```python
from build123d import *

# Parameters (mm, degrees)
SKETCH_1_W          = 100
SKETCH_1_H          = 100
EXTRUDE_1_DEPTH     = 2
SKETCH_2_W          = 6
SKETCH_2_H          = 12
EXTRUDE_2_DEPTH     = 10
SKETCH_3_R          = 3.725
CUT_EXTRUDE_1_DEPTH = 142.929559994
SKETCH_4_R          = 6
EXTRUDE_3_DEPTH     = 5
SKETCH_5_R          = 3.75
CUT_EXTRUDE_2_DEPTH = 142.594491418
SKETCH_6_W          = 100
SKETCH_6_H          = 19
CUT_EXTRUDE_3_DEPTH = 142.774468788
CUT_EXTRUDE_4_DEPTH = 130.077496102
FILLET_1_R          = 6
CUT_EXTRUDE_6_DEPTH = 130.077496102
FILLET_2_R          = 2
FILLET_3_R          = 2


# Some blends are built 0.0001 mm under size
with BuildPart() as part:
    # 草图1 → 凸台-拉伸1 (new body)
    with BuildSketch(Plane(origin=(0, 0, 0), x_dir=(1, 0, 0), z_dir=(0, 1, 0))):
        with Locations((50, -50)):
            Rectangle(SKETCH_1_W, SKETCH_1_H)
    extrude(amount=EXTRUDE_1_DEPTH)

    # 草图2 → 凸台-拉伸2 (add)
    with BuildSketch(Plane(origin=(0, 2, 0), x_dir=(1, 0, 0), z_dir=(0, 1, 0))):
        with Locations((97, -25)):
            Rectangle(SKETCH_2_W, SKETCH_2_H)
        with Locations((97, -75)):
            Rectangle(SKETCH_2_W, SKETCH_2_H)
    extrude(amount=EXTRUDE_2_DEPTH)

    # 草图3 → 切除-拉伸1 (cut, through all)
    with BuildSketch(Plane(origin=(100, 0, 0), x_dir=(0, 0, -1), z_dir=(1, 0, 0))):
        with Locations((-25, 6)):
            Circle(SKETCH_3_R)
        with Locations((-75, 6)):
            Circle(SKETCH_3_R)
    extrude(amount=-CUT_EXTRUDE_1_DEPTH, mode=Mode.SUBTRACT)

    # 草图4 → 凸台-拉伸3 (add)
    with BuildSketch(Plane(origin=(0, 2, 0), x_dir=(1, 0, 0), z_dir=(0, 1, 0))):
        with Locations(Location((50, -50, 0), (0, 0, 270))):
            Circle(SKETCH_4_R)
    extrude(amount=EXTRUDE_3_DEPTH)

    # 草图5 → 切除-拉伸2 (cut, through all)
    with BuildSketch(Plane(origin=(0, 7, 0), x_dir=(1, 0, 0), z_dir=(0, 1, 0))):
        with Locations(Location((50, -50, 0), (0, 0, 270))):
            Circle(SKETCH_5_R)
    extrude(amount=-CUT_EXTRUDE_2_DEPTH, mode=Mode.SUBTRACT)

    # 草图6 → 切除-拉伸3 (cut, through all)
    with BuildSketch(Plane(origin=(0, 2, 0), x_dir=(1, 0, 0), z_dir=(0, 1, 0))):
        with Locations((50, -90.5)):
            Rectangle(SKETCH_6_W, SKETCH_6_H)
        with Locations((50, -9.5)):
            Rectangle(SKETCH_6_W, SKETCH_6_H)
    extrude(amount=-CUT_EXTRUDE_3_DEPTH, mode=Mode.SUBTRACT)

    # 草图7 → 切除-拉伸4 (cut, through all)
    with BuildSketch(Plane(origin=(0, 2, 0), x_dir=(1, 0, 0), z_dir=(0, 1, 0))):
        with BuildLine():
            Line((55.73131114, -53.066279932), (94, -69))
            Line((94, -69), (94, -31))
            Line((94, -31), (55.73131114, -46.933720068))
            ThreePointArc((55.73131114, -46.933720068), (56.304899777, -48.41941821), (56.5, -50))
            ThreePointArc((56.5, -50), (56.304899777, -51.58058179), (55.73131114, -53.066279932))
        make_face()
        Polygon((0, -19), (53.212773637, -41.880071279), (94, -19), align=None)
        with BuildLine():
            Line((4, -75.253806127), (47.820913419, -56.123853499))
            ThreePointArc((47.820913419, -56.123853499), (43.5, -50), (47.820913419, -43.876146501))
            Line((47.820913419, -43.876146501), (4, -24.746193873))
            Line((4, -24.746193873), (4, -75.253806127))
        make_face()
        Polygon((94, -81), (53.212773637, -58.119928721), (0, -81), align=None)
    extrude(amount=-CUT_EXTRUDE_4_DEPTH, mode=Mode.SUBTRACT)

    # 圆角1
    fillet_1_edges = [part.edges().sort_by_distance(p)[0] for p in [
        (97, 12, 81),
        (97, 12, 69),
        (97, 12, 31),
        (97, 12, 19),
    ]]
    fillet(fillet_1_edges, radius=FILLET_1_R - 0.0001)  # a hair under: the kernel refuses the full size

    # 草图8 → 切除-拉伸6 (cut, through all)
    with BuildSketch(Plane(origin=(0, 2, 0), x_dir=(1, 0, 0), z_dir=(0, 1, 0))):
        Polygon((91.5, -23.268889447), (91.5, -29.332868234), (56.926900292, -43.727876504), (56.51218358, -42.895713945), align=None)
        Polygon((91.5, -70.667131766), (91.5, -76.731110553), (56.51218358, -57.104286055), (56.926900292, -56.272123496), align=None)
    extrude(amount=-CUT_EXTRUDE_6_DEPTH, mode=Mode.SUBTRACT)

    # 圆角2
    fillet_2_edges = [part.edges().sort_by_distance(p)[0] for p in [
        (47.820913419, 1, 43.876146501),
        (47.820913419, 1, 56.123853499),
        (55.73131114, 1, 53.066279932),
        (55.73131114, 1, 46.933720068),
    ]]
    fillet(fillet_2_edges, radius=FILLET_2_R)

    # 圆角3
    # the kernel refuses this fillet: 2 mm, written as the material it adds along each edge
    with BuildSketch(Plane(origin=(4, 2, 75.253806127), x_dir=(0, 0, -1), z_dir=(0, -1, 0)), Plane(origin=(4, 2, 24.746193873), x_dir=(0.9164772733710811, 0, 0.4000867498359684), z_dir=(0, -1, 0))) as fillet_3_piece_1:
        with BuildLine():
            CenterArc((FILLET_3_R * 1.52768299937, FILLET_3_R), FILLET_3_R, 156.416398259, 113.583601741)
            Line((FILLET_3_R * 0.611205725997, FILLET_3_R * 1.40008674984), (0, 0))
            Line((0, 0), (FILLET_3_R * 1.52768299937, 0))
        make_face()
    extrude(amount=2)
    with BuildSketch(Plane(origin=(53.212773637, 2, 58.119928721), x_dir=(-0.9186780925924477, 0, 0.39500704068497583), z_dir=(0, -1, 0))) as fillet_3_piece_2:
        with BuildLine():
            CenterArc((FILLET_3_R * 0.493765794488, -FILLET_3_R), FILLET_3_R, 90, 52.557168538)
            Line((-FILLET_3_R * 0.300194560291, -FILLET_3_R * 0.39203046537), (0, 0))
            Line((0, 0), (FILLET_3_R * 0.493765794488, 0))
        make_face()
    extrude(amount=2)
    with BuildSketch(Plane(origin=(53.212773637, 2, 41.880071279), x_dir=(-0.918678092592448, 0, -0.395007040684975), z_dir=(0, -1, 0))) as fillet_3_piece_3:
        with BuildLine():
            CenterArc((FILLET_3_R * 0.493765794488, FILLET_3_R), FILLET_3_R, 217.442831462, 52.557168538)
            Line((-FILLET_3_R * 0.300194560291, FILLET_3_R * 0.39203046537), (0, 0))
            Line((0, 0), (FILLET_3_R * 0.493765794488, 0))
        make_face()
    extrude(amount=2)
    with BuildSketch(Plane(origin=(91.5, 2, 23.268889447), x_dir=(-0.8721482225909527, 0, 0.48924173762204914), z_dir=(0, -1, 0))) as fillet_3_piece_4:
        with BuildLine():
            CenterArc((FILLET_3_R * 1.70755577899, -FILLET_3_R), FILLET_3_R, 90, 119.290755367)
            Line((FILLET_3_R * 0.8354075564, -FILLET_3_R * 1.48924173762), (0, 0))
            Line((0, 0), (FILLET_3_R * 1.70755577899, 0))
        make_face()
    extrude(amount=2)
    with BuildSketch(Plane(origin=(91.5, 2, 29.332868234), x_dir=(-0.9231759584436576, 0, 0.38437761348917576), z_dir=(0, -1, 0))) as fillet_3_piece_5:
        with BuildLine():
            CenterArc((FILLET_3_R * 0.666852706551, FILLET_3_R), FILLET_3_R, 202.605107184, 67.394892816)
            Line((-FILLET_3_R * 0.256323251893, FILLET_3_R * 0.615622386511), (0, 0))
            Line((0, 0), (FILLET_3_R * 0.666852706551, 0))
        make_face()
    extrude(amount=2)
    with BuildSketch(Plane(origin=(91.5, 2, 70.667131766), x_dir=(-0.923175958443657, 0, -0.38437761348917726), z_dir=(0, -1, 0))) as fillet_3_piece_6:
        with BuildLine():
            CenterArc((FILLET_3_R * 0.666852706551, -FILLET_3_R), FILLET_3_R, 90, 67.394892816)
            Line((-FILLET_3_R * 0.256323251893, -FILLET_3_R * 0.615622386511), (0, 0))
            Line((0, 0), (FILLET_3_R * 0.666852706551, 0))
        make_face()
    extrude(amount=2)
    with BuildSketch(Plane(origin=(91.5, 2, 76.731110553), x_dir=(-0.8721482225909533, 0, -0.4892417376220482), z_dir=(0, -1, 0))) as fillet_3_piece_7:
        with BuildLine():
            CenterArc((FILLET_3_R * 1.70755577899, FILLET_3_R), FILLET_3_R, 150.709244633, 119.290755367)
            Line((FILLET_3_R * 0.8354075564, FILLET_3_R * 1.48924173762), (0, 0))
            Line((0, 0), (FILLET_3_R * 1.70755577899, 0))
        make_face()
    extrude(amount=2)
    with BuildSketch(Plane(origin=(94, 2, 31), x_dir=(0, 0, 1), z_dir=(0, -1, 0)), Plane(origin=(94, 2, 69), x_dir=(-0.9231759584436573, 0, -0.3843776134891767), z_dir=(0, -1, 0))) as fillet_3_piece_8:
        with BuildLine():
            CenterArc((FILLET_3_R * 1.49958152704, FILLET_3_R), FILLET_3_R, 157.394892816, 112.605107184)
            Line((FILLET_3_R * 0.576405568596, FILLET_3_R * 1.38437761349), (0, 0))
            Line((0, 0), (FILLET_3_R * 1.49958152704, 0))
        make_face()
    extrude(amount=2)
    # the kernel refuses this fillet: 2 mm, written as the material it takes off along each edge
    with BuildSketch(Plane(origin=(0, 9.592469288, 81), x_dir=(0.9186780925924475, 0, -0.3950070406849762), z_dir=(0, -1, 0)), Plane(origin=(0, 9.592469288, 19), x_dir=(0, 0, 1), z_dir=(0, -1, 0))) as fillet_3_2_piece_1:
        with BuildLine():
            CenterArc((FILLET_3_R * 1.51849385757, -FILLET_3_R), FILLET_3_R, 90, 113.266413172)
            Line((FILLET_3_R * 0.599815764977, -FILLET_3_R * 1.39500704068), (0, 0))
            Line((0, 0), (FILLET_3_R * 1.51849385757, 0))
        make_face()
    extrude(amount=17.184938576, mode=Mode.SUBTRACT)


solid = part.part
```
Work out the finished part from the listing and answer in its coordinate system (mm). A direction names the side the tool comes from. Give positions to 0.01 mm unless a question says otherwise; leave off trailing zeros. Loops run counter-clockwise (first coordinate to the right, second up) from the corner with the lowest first, then second, coordinate; pieces in that order, holes last. Notation, with made-up numbers: (49, -17.75) -> (89, -17.75) arc R28 ccw to (89, 15.25) -> close; hole circle Ø4 at (-11.75, 71). An arc over 180 degrees is marked (long way). Put each result on its own line as item: value. Start each with the question number.
Item 1: Each of these flat-tipped pins is pushed along its axis until it touches: P1, Ø10, axis at x = 22, z = 28.5, coming from the +Y side; P2, Ø6.5, axis at y = 6, z = 75, coming from the +X side; P3, Ø13, axis at x = 49, z = 52, coming from the +Y side; P4, Ø12, axis at x = 50, z = 50, coming from the -Y side. Where does it stop, or does it pass through?
Item 2: Find the intervals of material crossed by L1, parallel to X at y = 5.25, z = 50; L2, parallel to Y at x = 98.35, z = 75 (3 decimals); L3, parallel to X at y = 1.75, z = 67.5, in increasing order. Write a range as [from, to].
Item 3: The part is cut by section D-D (x = 27). Give the vertices of the cut face in (y, z), then the cut area to 3 significant figures.
Item 4: The part is cut by section B-B (y = 10.75). Give the vertices of the cut face in (x, z), then the cut area to 3 significant figures.
Item 5: The mould has two halves that part along X. Classify faces 1 (the face through (50, 4, 44)), 2 (the face through (27.89, 1.01, 69.01)), 3 (the face through (57, 2, 46)): released by +X, released by -X, zero draft, split by the parting line, or undercut.
Item 6: Which of the six approach directions +Z, -Z, +X, -X, +Y, -Y give full straight-line access (tool end or side, diameter ignored) to faces 4 (the face through (45.673, 0.986, 56.173)), 5 (the face through (94, 10, 25)), 6 (the face through (97, 4, 69))?
Item 7: The part is cut by section A-A (x = 48.5). Give the vertices of the cut face in (y, z), then the cut area to 3 significant figures.
Item 8: The part is cut by section C-C (x = 59). Give the vertices of the cut face in (y, z), then the cut area to 3 significant figures.
Answers below:
1. P1: y = 2
1. P2: through
1. P3: y = 7
1. P4: y = 0
2. L1: [44, 46.25], [53.75, 56]
2. L2: [0, 2.275], [9.725, 12]
2. L3: [0, 4], [21.76, 31.4], [69.93, 75.04], [83.89, 90.4], [93.32, 100]
3. outline: (0, 30.61) -> (2, 30.61) -> (2, 34.79) -> (0, 34.79) -> close; (0, 65.21) -> (2, 65.21) -> (2, 69.39) -> (0, 69.39) -> close
3. area: 16.7 mm2
4. outline: (94, 21.33) -> (100, 21.33) -> (100, 28.67) -> (94, 28.67) -> close; (94, 71.33) -> (100, 71.33) -> (100, 78.67) -> (94, 78.67) -> close
4. area: 88.0 mm2
5. face 1: split by the parting line
5. face 2: undercut
5. face 3: zero draft
6. face 4: +Y, -Y
6. face 5: +Z, -Z, -X, +Y
6. face 6: +X, -X, +Y
7. outline: (0, 39.85) -> (2, 39.85) -> (2, 44.19) -> (7, 44.19) -> (7, 46.56) -> (0, 46.56) -> close; (0, 53.44) -> (7, 53.44) -> (7, 55.81) -> (2, 55.81) -> (2, 60.15) -> (0, 60.15) -> close
7. area: 50.6 mm2
8. outline: (0, 38.63) -> (2, 38.63) -> (2, 41.5) -> (0, 41.5) -> close; (0, 42.86) -> (2, 42.86) -> (2, 45.57) -> (0, 45.57) -> close; (0, 54.43) -> (2, 54.43) -> (2, 57.14) -> (0, 57.14) -> close; (0, 58.5) -> (2, 58.5) -> (2, 61.37) -> (0, 61.37) -> close
8. area: 22.3 mm2
